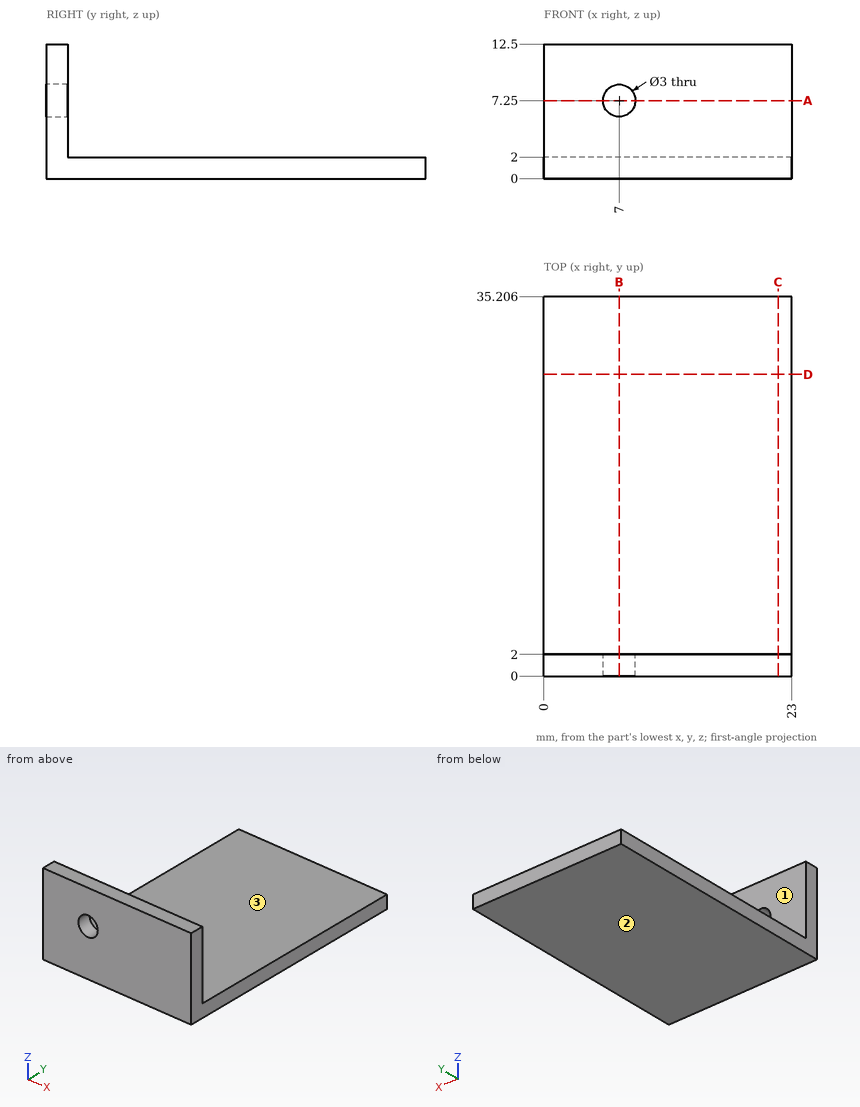
For this review, use the dimensioned drawing (mm, ordinates from the lowest corner) and the shaded views. Coordinates: 2 decimals unless noted, no trailing zeros. Write each loop counter-clockwise with the first axis right and the second up, starting at its lowest first coordinate (ties: lowest second). Pieces come first, ordered by that corner, then holes. Notation, with made-up numbers: (-30, 42.5) - (6, 42.5) arc R25 cw to (6, 57.5) - close; hole circle Ø9 at (45.25, -34.5). An arc over 180 degrees is marked (long way). Answer in a Markdown table with one row per item. Add a question column.
Q1. Consider section A-A on z = 7.25. Give the boundary of the cut face in (x, y).
Q2. To check wall thickness, follow line 1 along X through (y, z) = (0.5, 7.25); line 2 along Y through (x, z) = (14, 3.5). State the ranges of each line that lie inside material, in increasing order. Write a range as from..to.
Q3. Consider section D-D on y = 28. Give the boundary of the cut face in (x, z).
Q4. Consider section B-B on x = 7. Give the boundary of the cut face in (y, z).
Q5. Consider section C-C on x = 21.75. Give the boundary of the cut face in (y, z).
Q6. Draft analysis for pull direction Z (two halves, no side actions). For the marked faces 1, 2 and 3, state which applies: +Z half, -Z half, draft (parallel to the pull), parting line (faces both ways), or undercut.
Q7. Clearance check with flat-ended pins moving along their axes: pin 1 (1 mm diameter, centred on x = 17, z = 4, fed in from -Y); pin 2 (5 mm diameter, centred on x = 9.5, z = 7, fed in from +Y); pin 3 (5 mm diameter, centred on x = 6.5, y = 28.5, fed in from +Z). State where each tip first meets the part, or that it passes through.
Answers below:
| question | item | result |
|---|---|---|
| 1 | outline | (0, 0) - (5.5, 0) - (5.5, 2) - (0, 2) - close; (8.5, 0) - (23, 0) - (23, 2) - (8.5, 2) - close |
| 2 | line 1 | 0..5.5, 8.5..23 |
| 2 | line 2 | 0..2 |
| 3 | outline | (0, 0) - (23, 0) - (23, 2) - (0, 2) - close |
| 4 | outline | (0, 0) - (35.21, 0) - (35.21, 2) - (2, 2) - (2, 5.75) - (0, 5.75) - close; (0, 8.75) - (2, 8.75) - (2, 12.5) - (0, 12.5) - close |
| 5 | outline | (0, 0) - (35.21, 0) - (35.21, 2) - (2, 2) - (2, 12.5) - (0, 12.5) - close |
| 6 | face 1 | draft |
| 6 | face 2 | -Z half |
| 6 | face 3 | +Z half |
| 7 | pin 1 | y = 0 |
| 7 | pin 2 | y = 2 |
| 7 | pin 3 | z = 2 |
